Read the model definition and answer for the solid it produces. Units are mm, in the model's axes. A direction names the side the tool comes from. Round coordinates to 2 decimals unless told otherwise and drop trailing zeros. Write each loop counter-clockwise with the first axis right and the second up, starting at its lowest first coordinate (ties: lowest second). Pieces come first, ordered by that corner, then holes. Notation, with made-up numbers: (6.25, 18.25) -> (44.25, 18.25) arc R12 ccw to (44.25, 24.25) -> close; hole circle Ø1 at (82.25, 12). An arc over 180 degrees is marked (long way). Return JSON: item names as keys, results as strings.
from build123d import *

# Parameters (mm, degrees)
SKETCH2_W          = 22
SKETCH2_H          = 28
SKETCH2_R          = 1.3
MAINBODY_DEPTH     = 2
SKETCH3_W          = 5
SKETCH3_H          = 5
CHIP_DEPTH         = 1
SKETCH4_R          = 0.695578212
CUT_EXTRUDE1_DEPTH = 18.916472867


with BuildPart() as part:
    # Sketch2 → MainBody (new body)
    with BuildSketch(Plane(origin=(0, 0, 0), x_dir=(1, 0, 0), z_dir=(0, 1, 0))):
        Rectangle(SKETCH2_W, SKETCH2_H)
        with Locations(Location((9, -1, 0), (0, 0, 270))):
            Circle(SKETCH2_R, mode=Mode.SUBTRACT)
        with Locations(Location((-9, -1, 0), (0, 0, 270))):
            Circle(SKETCH2_R, mode=Mode.SUBTRACT)
        with Locations(Location((-9, -12, 0), (0, 0, 270))):
            Circle(SKETCH2_R, mode=Mode.SUBTRACT)
        with Locations(Location((9, -12, 0), (0, 0, 270))):
            Circle(SKETCH2_R, mode=Mode.SUBTRACT)
    extrude(amount=MAINBODY_DEPTH)

    # Sketch3 → chip (add)
    with BuildSketch(Plane(origin=(0, 2, 0), x_dir=(1, 0, 0), z_dir=(0, 1, 0))):
        with Locations((0, -6.5)):
            Rectangle(SKETCH3_W, SKETCH3_H)
    extrude(amount=CHIP_DEPTH)

    # Sketch4 → Cut-Extrude1 (cut, through all)
    with BuildSketch(Plane(origin=(0, 2, 0), x_dir=(1, 0, 0), z_dir=(0, 1, 0))):
        with Locations(Location((-8.137841022, 11.921007347, 0), (0, 0, 270))):
            Circle(SKETCH4_R)
        with Locations(Location((8.5, 12, 0), (0, 0, 270))):
            Circle(SKETCH4_R)
        with Locations(Location((-5.737841022, 11.921007347, 0), (0, 0, 270))):
            Circle(SKETCH4_R)
        with Locations(Location((-3.337841022, 11.921007347, 0), (0, 0, 270))):
            Circle(SKETCH4_R)
        with Locations(Location((-0.937841022, 11.921007347, 0), (0, 0, 270))):
            Circle(SKETCH4_R)
        with Locations(Location((1.462158978, 11.921007347, 0), (0, 0, 270))):
            Circle(SKETCH4_R)
        with Locations(Location((3.862158978, 11.921007347, 0), (0, 0, 270))):
            Circle(SKETCH4_R)
        with Locations(Location((6.262158978, 11.921007347, 0), (0, 0, 270))):
            Circle(SKETCH4_R)
    extrude(amount=-CUT_EXTRUDE1_DEPTH, mode=Mode.SUBTRACT)


solid = part.part
Item 1: Flat-ended cylindrical pins translate along their axes: pin 1 (1.6 mm diameter, centred on x = 6.26, z = -11.92, fed in from +Y); pin 2 (0.8 mm diameter, centred on y = 2.5, z = 7, fed in from -X); pin 3 (0.5 mm diameter, centred on x = 1, y = 2.5, fed in from -Z). Find the tip coordinate at first contact, or state that the pin passes through.
Worked answers:
{"pin 1": "stops at y = 2", "pin 2": "stops at x = -2.5", "pin 3": "stops at z = 4"}
Item 2: A tool of negligible diameter and unlimited length cuts with its end or side. For faces 4 (the flat face through (0, 2.5, 4)), 5 (the flat face through (-2.5, 2.5, 6.5)), 6 (the flat face through (2.5, 2.5, 6.5)), 7 (the flat face through (0, 2.5, 9)), from which of +Z, -Z, +X, -X, +Y, -Y can it reach the whole face along a straight path? Write none if from no direction.
Worked answers:
{"face 4": "-Z, +X, -X, +Y", "face 5": "+Z, -Z, -X, +Y", "face 6": "+Z, -Z, +X, +Y", "face 7": "+Z, +X, -X, +Y"}
Item 3: Section D-D (z = 2) is taken. Give the vertices of the cut face in (x, y), then the cut area to 3 significant figures.
Worked answers:
{"outline": "(-11, 0) -> (-9.83, 0) -> (-9.83, 2) -> (-11, 2) -> close; (-8.17, 0) -> (8.17, 0) -> (8.17, 2) -> (-8.17, 2) -> close; (9.83, 0) -> (11, 0) -> (11, 2) -> (9.83, 2) -> close", "area": "37.4 mm2"}
Item 4: Straight lines are drawn through the part: L1, parallel to X at y = 1.35, z = 12; L2, parallel to Z at x = -8, y = 0.95; L3, parallel to Y at x = 7.75, z = -3.25. For each, find the intervals that lie inside material, in ascending order. Write a range as [from, to].
Worked answers:
{"L1": "x = [-11, -10.3], [-7.7, 7.7], [10.3, 11]", "L2": "z = [-14, -12.6], [-11.24, 0.17], [1.83, 11.17], [12.83, 14]", "L3": "y = [0, 2]"}
Item 5: Section B-B (y = 1.55) is taken. State how many separate pieces and enclosed holes the cut face has, then the cut area to 3 significant figures.
Worked answers:
{"separate pieces": "1", "enclosed holes": "12", "area": "583 mm2"}
Item 6: Section A-A (z = 12) is taken. Give the vertices of the cut face in (x, y), then the cut area to 3 significant figures.
Worked answers:
{"outline": "(-11, 0) -> (-10.3, 0) -> (-10.3, 2) -> (-11, 2) -> close; (-7.7, 0) -> (7.7, 0) -> (7.7, 2) -> (-7.7, 2) -> close; (10.3, 0) -> (11, 0) -> (11, 2) -> (10.3, 2) -> close", "area": "33.6 mm2"}
Item 7: Section C-C (z = -6.25) is taken. Give the vertices of the cut face in (x, y), then the cut area to 3 significant figures.
Worked answers:
{"outline": "(-11, 0) -> (11, 0) -> (11, 2) -> (-11, 2) -> close", "area": "44.0 mm2"}
Item 8: For a pull along Z with two mould halves and no side action, classify faces 1 (the flat face through (0, 1, 14)), 2 (the flat face through (0, 3, 6)), 3 (the cylindrical face through (10.29, 0.99, 0.83)) as released by +Z, released by -Z, zero draft, split by the parting line, or undercut.
Worked answers:
{"face 1": "released by +Z", "face 2": "zero draft", "face 3": "undercut"}
